Verification items for this drawing (mm, ordinates from the low corner). Coordinates: 2 decimals unless noted, no trailing zeros. Order: outer loops, then holes, each group sorted by start corner. A loop starts at its lowest first (then second) coordinate and runs counter-clockwise, first axis right, second up. Notation, with made-up numbers: M 53,59 L 58,59 A32 cw 58,88 Z; hole C 59.5,-30 d2. An arc over 180 degrees is marked long. Return JSON: item names as keys, results as strings. Group by question number.
1. Section check B-B, the plane y = 78. Record the cut outline in (x, z).
2. Material ranges on line 1 along X through (y, z) = (93, 2.15); line 2 along Y through (x, z) = (21.25, 2.25); line 3 along Y through (x, z) = (5.5, 2.55), recorded low to high.
3. Section check A-A, the plane x = 6.25. Record the cut outline in (y, z).
4. Section check C-C, the plane z = 0.95. Record the cut outline in (x, y), plus the area to 3 significant figures.
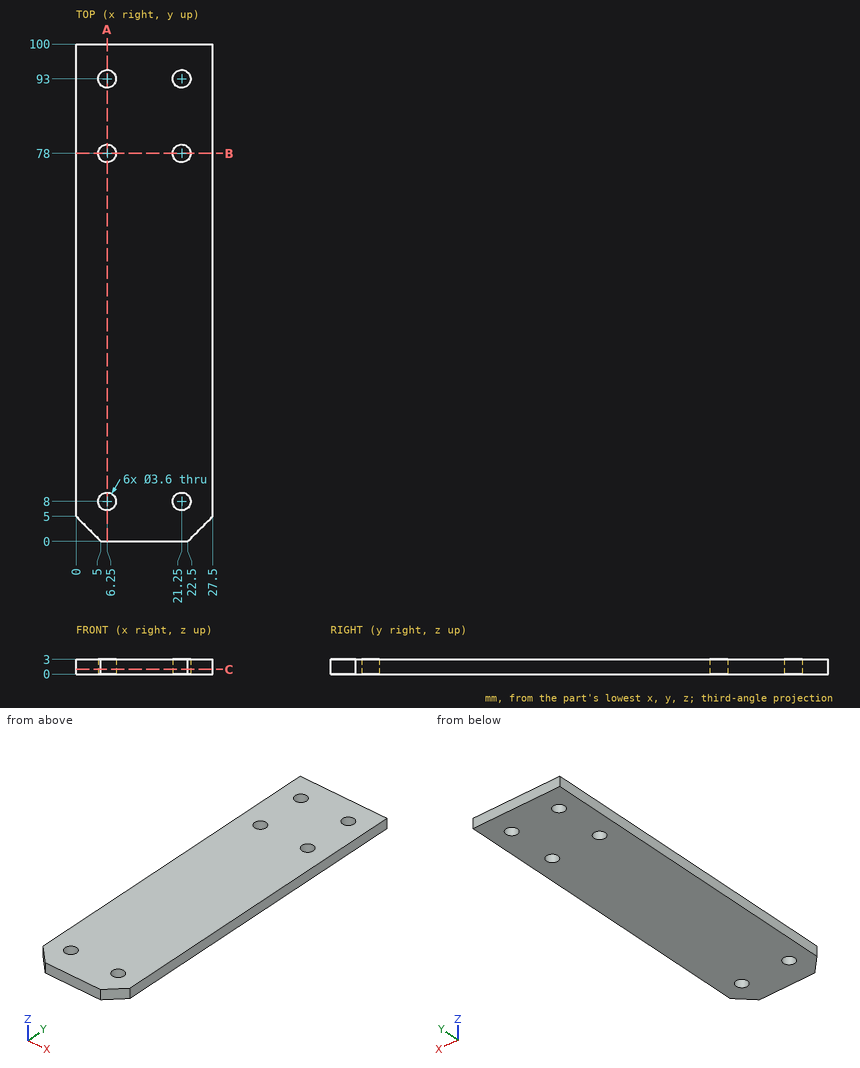
Answers follow:
{
 "1": {"outline": "M 0,0 L 4.45,0 L 4.45,3 L 0,3 Z; M 8.05,0 L 19.45,0 L 19.45,3 L 8.05,3 Z; M 23.05,0 L 27.5,0 L 27.5,3 L 23.05,3 Z"},
 "2": {"line 1": "0 to 4.45, 8.05 to 19.45, 23.05 to 27.5", "line 2": "0 to 6.2, 9.8 to 76.2, 79.8 to 91.2, 94.8 to 100", "line 3": "0 to 6.36, 9.64 to 76.36, 79.64 to 91.36, 94.64 to 100"},
 "3": {"outline": "M 0,0 L 6.2,0 L 6.2,3 L 0,3 Z; M 9.8,0 L 76.2,0 L 76.2,3 L 9.8,3 Z; M 79.8,0 L 91.2,0 L 91.2,3 L 79.8,3 Z; M 94.8,0 L 100,0 L 100,3 L 94.8,3 Z"},
 "4": {"outline": "M 0,5 L 5,0 L 22.5,0 L 27.5,5 L 27.5,100 L 0,100 Z; hole C 6.25,8 d3.6; hole C 6.25,78 d3.6; hole C 6.25,93 d3.6; hole C 21.25,8 d3.6; hole C 21.25,78 d3.6; hole C 21.25,93 d3.6", "area": "2,660 mm^2"}
}
